```python
from build123d import *

# Parameters (mm, degrees)
SKETCH1_W           = 23
SKETCH1_H           = 23
BOSS_EXTRUDE1_DEPTH = 600
SKETCH2_R           = 4.25
CUT_EXTRUDE1_DEPTH  = 350
SKETCH3_R           = 5.25
CUT_EXTRUDE2_DEPTH  = 49
FILLET1_R           = 0.5


with BuildPart() as part:
    # Sketch1 → Boss-Extrude1 (new body)
    with BuildSketch(Plane(origin=(0, 0, 0), x_dir=(1, 0, 0), z_dir=(0, 1, 0))):
        with Locations((11.5, 11.5)):
            Rectangle(SKETCH1_W, SKETCH1_H)
    extrude(amount=BOSS_EXTRUDE1_DEPTH)

    # Sketch2 → Cut-Extrude1 (cut)
    with BuildSketch(Plane(origin=(23, 0, 0), x_dir=(0, 0, -1), z_dir=(1, 0, 0))):
        with Locations((11.5, 20)):
            Circle(SKETCH2_R)
    extrude(amount=-CUT_EXTRUDE1_DEPTH, mode=Mode.SUBTRACT)

    # Sketch3 → Cut-Extrude2 (cut)
    with BuildSketch(Plane(origin=(23, 0, 0), x_dir=(0, 0, -1), z_dir=(1, 0, 0))):
        with Locations((11.5, 590)):
            Circle(SKETCH3_R)
    extrude(amount=-CUT_EXTRUDE2_DEPTH, mode=Mode.SUBTRACT)

    # Fillet1
    fillet1_edges = [part.edges().sort_by_distance(p)[0] for p in [
        (23, 600, -11.5),
        (11.5, 600, -23),
        (0, 20, -7.25),
        (23, 20, -7.25),
        (0, 590, -6.25),
        (23, 590, -6.25),
        (0, 600, -11.5),
        (11.5, 0, -23),
        (23, 0, -11.5),
        (11.5, 0, 0),
        (0, 0, -11.5),
        (11.5, 600, 0),
        (0, 300, -23),
        (23, 300, -23),
        (23, 300, 0),
        (0, 300, 0),
    ]]
    fillet(fillet1_edges, radius=FILLET1_R)


solid = part.part
```
Read the model definition and answer for the solid it produces. Units are mm, in the model's axes. Give positions to 0.01 mm unless a question says otherwise; leave off trailing zeros. Write each loop counter-clockwise with the first axis right and the second up, starting at its lowest first coordinate (ties: lowest second). Pieces come first, ordered by that corner, then holes. Notation, with made-up numbers: (5, 35.25) - (26, 35.25) arc R27 ccw to (26, 52.25) - close; hole circle Ø11 at (57.5, 4.5). An arc over 180 degrees is marked (long way). Write item = value, one per line. Start each with the question number.
Item 1: The mould has two halves that part along Z. Classify faces 1 (the flat face through (11, 296, -23)), 2 (the cylindrical face through (11.654, 584.875, -10.362)), 3 (the flat face through (0, 296, -11)), 4 (the flat face through (11, 296, 0)): +Z half, -Z half, draft (parallel to the pull), parting line (faces both ways), or undercut.
Item 2: Find the intervals of material crossed by probe 1 along Y at (x, z) = (5.75, -11.5); probe 2 along Y at (x, z) = (9.5, -13.25); probe 3 along Z at (x, y) = (7.5, 590), in increasing order. Write a range as [from, to].
Item 3: Find section A-A (z = -11.5). Give the vertices of the cut face in (x, y), then the cut area to 3 significant figures.
Response:
q1.face_1 = -Z half
q1.face_2 = undercut
q1.face_3 = draft
q1.face_4 = +Z half
q2.probe_1 = [0, 15.75], [24.25, 584.75], [595.25, 600]
q2.probe_2 = [0, 16.13], [23.87, 585.05], [594.95, 600]
q2.probe_3 = [-23, -16.75], [-6.25, 0]
q3.outline = (0, 0.5) arc R0.5 ccw to (0.5, 0) - (22.5, 0) arc R0.5 ccw to (23, 0.5) - (23, 15.25) arc R0.5 ccw to (22.5, 15.75) - (0.5, 15.75) arc R0.5 ccw to (0, 15.25) - close; (0, 24.75) arc R0.5 ccw to (0.5, 24.25) - (22.5, 24.25) arc R0.5 ccw to (23, 24.75) - (23, 584.25) arc R0.5 ccw to (22.5, 584.75) - (0.5, 584.75) arc R0.5 ccw to (0, 584.25) - close; (0, 595.75) arc R0.5 ccw to (0.5, 595.25) - (22.5, 595.25) arc R0.5 ccw to (23, 595.75) - (23, 599.5) arc R0.5 ccw to (22.5, 600) - (0.5, 600) arc R0.5 ccw to (0, 599.5) - close
q3.area = 13,400 mm²
